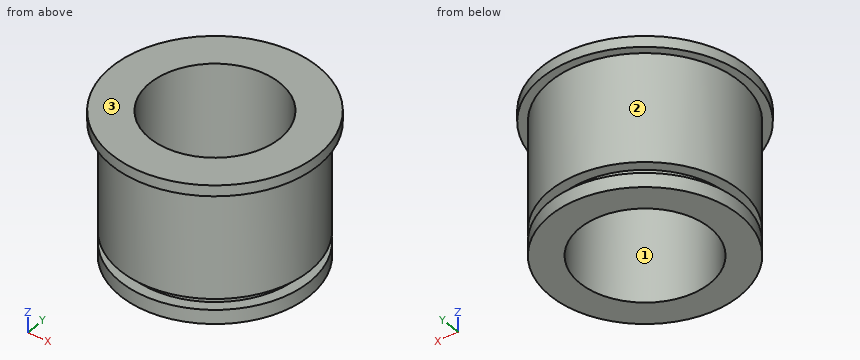
from build123d import *

# Parameters (mm, degrees)
F0_R     = 8.73125
F0_R_2   = 6
F1_DEPTH = 12.3
F2_R     = 9.525
F2_R_2   = 6
F3_DEPTH = 1
F4_W     = 2
F4_H     = 1


with BuildPart() as f1:
    # F0 (on Top) → F1 (new body)
    with BuildSketch(Plane.XY):
        Circle(F0_R)
        Circle(F0_R_2, mode=Mode.SUBTRACT)
    extrude(amount=F1_DEPTH)

    # F2 (on face) → F3 (join)
    with BuildSketch(Plane.XY.offset(12.3)):
        Circle(F2_R)
        Circle(F2_R_2, mode=Mode.SUBTRACT)
    extrude(amount=F3_DEPTH)

    # F4 (on Front) → F5 (revolve, cut)
    with BuildSketch(Plane.XZ):
        with Locations((-8.73125, 1.8)):
            Rectangle(F4_W, F4_H)
    revolve(axis=Axis((0, 0, 7.145868), (0, 0, -1)), mode=Mode.SUBTRACT)


solid = f1.part
Build history of the part. All positions in model axes, mm. Face numbers are marked on the shaded views. Coordinates: 2 decimals unless noted, no trailing zeros. Order: outer loops, then holes, each group sorted by start corner. A loop starts at its lowest first (then second) coordinate and runs counter-clockwise, first axis right, second up. Notation, with made-up numbers: (-2, 80.5) - (38, 80.5) arc R27 cw to (38, 118.5) - close; hole circle Ø3 at (84.25, 20.5). An arc over 180 degrees is marked (long way). Write each question's results on one line, items separated by ' | '. Start each with the question number.
Item 1: Band-saw the part on D-D on y = -8. Write the cut outline in (x, z).
Item 2: Flat gauge pins, fed straight in: pin 1 (5 mm diameter, centred on x = 7, z = 6.5, fed in from +Y); pin 2 (3 mm diameter, centred on x = 1.5, z = 6, fed in from +Y); pin 3 (6 mm diameter, centred on x = 6.5, z = 6, fed in from -Y). Where does each tip first touch, or does it go through?
Item 3: Wall check: probe 1 along Y at (x, z) = (0, 7); probe 2 along Z at (x, y) = (8, -2.5); probe 3 along X at (y, z) = (0.75, 1.5). Give the ranges that are in metal, low to high. Write a range as [from, to].
Item 4: Mould opens along Y. For the marked faces 1, 2 and 3 say: released by +Y, released by -Y, zero draft, split by the parting line, or undercut.
Item 5: Band-saw the part on A-A on y = 0. Write the cut outline in (x, z) (3 decimals).
Item 6: Band-saw the part on C-C on z = 7.75. Write the cut outline in (x, y).
Numbers:
1) outline: (-5.17, 12.3) - (-3.5, 12.3) - (-3.5, 2.3) - (3.5, 2.3) - (3.5, 12.3) - (5.17, 12.3) - (5.17, 13.3) - (-5.17, 13.3) - close; (-3.5, 0) - (3.5, 0) - (3.5, 1.3) - (-3.5, 1.3) - close
2) pin 1: y = 7.48 | pin 2: y = 8.73 | pin 3: y = -8
3) probe 1: [-8.73, -6], [6, 8.73] | probe 2: [0, 1.3], [2.3, 13.3] | probe 3: [-7.69, -5.95], [5.95, 7.69]
4) face 1: undercut | face 2: split by the parting line | face 3: zero draft
5) outline: (-9.525, 12.3) - (-8.731, 12.3) - (-8.731, 2.3) - (-7.731, 2.3) - (-7.731, 1.3) - (-8.731, 1.3) - (-8.731, 0) - (-6, 0) - (-6, 13.3) - (-9.525, 13.3) - close; (6, 0) - (8.731, 0) - (8.731, 1.3) - (7.731, 1.3) - (7.731, 2.3) - (8.731, 2.3) - (8.731, 12.3) - (9.525, 12.3) - (9.525, 13.3) - (6, 13.3) - close
6) outline: circle Ø17.46 at (0, 0); hole circle Ø12 at (0, 0)
